Geometry check sheet. Reference: the model listing, model coordinates, mm. A direction names the side the tool comes from. Round coordinates to 2 decimals unless told otherwise and drop trailing zeros. Order: outer loops, then holes, each group sorted by start corner. A loop starts at its lowest first (then second) coordinate and runs counter-clockwise, first axis right, second up. Notation, with made-up numbers: (-28.75, 88) -> (14.25, 88) arc R8 cw to (14.25, 98) -> close; hole circle Ø5 at (57.5, 19). An arc over 180 degrees is marked (long way). Use a Markdown table: item, result. Add a question column.
Item 1: Sectioned sample at B-B, the plane y = 5.5. Record the cut outline in (x, z), and give its area (3 significant figures).
Item 2: Gauge pin test, flat ends, axial feed: pin 1 Ø5 at (y, z) = (7.5, -24) entering from +X; pin 2 Ø3 at (y, z) = (3.5, 13.5) entering from -X; pin 3 Ø12 at (x, z) = (-2, -28.5) entering from +Y; pin 4 Ø1.5 at (x, z) = (-25.5, -38) entering from -Y. Record the tip position at first contact, or that the pin passes through.
Item 3: Material ranges on probe 1 along X at (y, z) = (2.25, -39.5); probe 2 along Y at (x, z) = (-28, 11); probe 3 along Z at (x, y) = (-30.5, -5.75), recorded low to high. Write a range as [from, to].
Item 4: Sectioned sample at A-A, the plane x = -9. Record the cut outline in (y, z), and give its area (3 significant figures).
Item 5: Sectioned sample at C-C, the plane x = 19. Record the cut outline in (y, z), and give its area (3 significant figures).
Item 6: Set-up check for faces 1 (the flat face through (-9, -3, 17.835)), 2 (the flat face through (-9, 7, 17.835)), 3 (the cylindrical face through (-10.36, 6.45, -45.91)): record each of +Z, -Z, +X, -X, +Y, -Y from which the full face is reachable in a straight line by a thin tool's end or side.
Item 7: Mould release check, pull along X, two halves, no side actions. Record for faces 4 (the cylindrical face through (-10.752, 6.451, -48.886)), 5 (the flat face through (-48.929, 1, 19)), 6 (the cylindrical face through (-9.58, 1.521, -39.962)): pulls with the +X half, pulls with the -X half, needs draft (parallel to the pull), parting line crosses it, or undercut.
Item 8: Sectioned sample at D-D, the plane y = -3. Record the cut outline in (x, z), and give its area (3 significant figures).
from build123d import *

# Parameters (mm, degrees)
BOSS_EXTRUDE1_DEPTH = 3
SKETCH2_R           = 14
SKETCH2_R_2         = 11
BOSS_EXTRUDE2_DEPTH = 7
SKETCH3_W           = 80
SKETCH3_H           = 17
BOSS_EXTRUDE3_DEPTH = 3
SKETCH5_R           = 5
CUT_EXTRUDE1_DEPTH  = 10


with BuildPart() as part:
    # Sketch1 → Boss-Extrude1 (new body)
    with BuildSketch(Plane(origin=(0, 0, 0), x_dir=(1, 0, 0), z_dir=(0, 1, 0))):
        with BuildLine():
            Line((-48.929144451, -17.835062273), (31.070855549, -17.835062273))
            Line((31.070855549, -17.835062273), (6.985518971, 43.196988966))
            ThreePointArc((6.985518971, 43.196988966), (-8.929144451, 52.904273338), (-24.843807874, 43.196988966))
            Line((-24.843807874, 43.196988966), (-48.929144451, -17.835062273))
        make_face()
    extrude(amount=BOSS_EXTRUDE1_DEPTH)

    # Sketch2 → Boss-Extrude2 (add)
    with BuildSketch(Plane(origin=(0, 3, 0), x_dir=(1, 0, 0), z_dir=(0, 1, 0))):
        with Locations((-8.929144451, 35.004937727)):
            Circle(SKETCH2_R)
        with Locations((-8.929144451, 35.004937727)):
            Circle(SKETCH2_R_2, mode=Mode.SUBTRACT)
    extrude(amount=BOSS_EXTRUDE2_DEPTH)

    # Sketch3 → Boss-Extrude3 (add)
    with BuildSketch(Plane.XY.offset(17.835062273)):
        with Locations((-8.929144451, 1.5)):
            Rectangle(SKETCH3_W, SKETCH3_H)
    extrude(amount=BOSS_EXTRUDE3_DEPTH)

    # Sketch5 → Cut-Extrude1 (cut)
    with BuildSketch(Plane(origin=(0, 3, 0), x_dir=(1, 0, 0), z_dir=(0, 1, 0))):
        with Locations((-8.929144451, 35.004937727)):
            Circle(SKETCH5_R)
    extrude(amount=-CUT_EXTRUDE1_DEPTH, mode=Mode.SUBTRACT)


solid = part.part
Found:
| question | item | result |
|---|---|---|
| 1 | outline | (-48.93, 17.84) -> (31.07, 17.84) -> (31.07, 20.84) -> (-48.93, 20.84) -> close; circle Ø28 at (-8.93, -35); hole circle Ø22 at (-8.93, -35) |
| 1 | area | 476 mm2 |
| 2 | pin 1 | stops at x = 2.19 |
| 2 | pin 2 | stops at x = -47.78 |
| 2 | pin 3 | stops at y = 10 |
| 2 | pin 4 | stops at y = 0 |
| 3 | probe 1 | x = [-26.3, -11.12], [-6.74, 8.44] |
| 3 | probe 2 | y = [0, 3] |
| 3 | probe 3 | z = [17.84, 20.84] |
| 4 | outline | (-7, 17.84) -> (0, 17.84) -> (0, -30.01) -> (3, -30.01) -> (3, -24.01) -> (10, -24.01) -> (10, -21.01) -> (3, -21.01) -> (3, 17.84) -> (10, 17.84) -> (10, 20.84) -> (-7, 20.84) -> close; (0, -52.9) -> (3, -52.9) -> (3, -49) -> (10, -49) -> (10, -46) -> (3, -46) -> (3, -40) -> (0, -40) -> close |
| 4 | area | 275 mm2 |
| 5 | outline | (-7, 17.84) -> (0, 17.84) -> (0, -12.75) -> (3, -12.75) -> (3, 17.84) -> (10, 17.84) -> (10, 20.84) -> (-7, 20.84) -> close |
| 5 | area | 143 mm2 |
| 6 | face 1 | -Z, +X, -X, -Y |
| 6 | face 2 | +X, -X, +Y |
| 6 | face 3 | +Y |
| 7 | face 4 | parting line crosses it |
| 7 | face 5 | pulls with the -X half |
| 7 | face 6 | undercut |
| 8 | outline | (-48.93, 17.84) -> (31.07, 17.84) -> (31.07, 20.84) -> (-48.93, 20.84) -> close |
| 8 | area | 240 mm2 |
